Geometry check sheet. Reference: the model listing, model coordinates, mm. A direction names the side the tool comes from. Coordinates: 2 decimals unless noted, no trailing zeros. Write each loop counter-clockwise with the first axis right and the second up, starting at its lowest first coordinate (ties: lowest second). Pieces come first, ordered by that corner, then holes. Notation, with made-up numbers: (76.5, 87) -> (129.5, 87) arc R21 cw to (129.5, 124) -> close; hole circle Ø8 at (-22, 10.25). An arc over 180 degrees is marked (long way). Put each result on its own line as item: value. Start each with the question number.
from build123d import *

# Parameters (mm, degrees)
F0_W      = 15
F0_H      = 63
F1_DEPTH  = 40
F4_W      = 15
F4_H      = 60
F2_W      = 45
F2_H      = 80
F1_FACE_W = 45
F1_FACE_H = 80
F8_W      = 30
F8_H      = 30
F9_DEPTH  = 50


with BuildPart() as f1:
    # F0 (on Front) → F1 (new body, symmetric)
    with BuildSketch(Plane.XZ):
        Polygon((-52.5, -6), (52.5, -6), (52.5, 6), (37.5, 6), (-52.5, 6), align=None)
        with Locations((45, 37.5)):
            Rectangle(F0_W, F0_H)
    extrude(amount=F1_DEPTH, both=True)

    # F4 (on offset) → F5 section 0
    with BuildSketch(Plane.XY.offset(52)):
        with Locations((-27, 0)):
            Rectangle(F4_W, F4_H)
    # F2 (on face) → F5 section 1
    with BuildSketch(Plane.XY.offset(6)):
        with Locations((-30, 0)):
            Rectangle(F2_W, F2_H)
    loft()

    # F4 (on offset) → F6 section 0
    with BuildSketch(Plane.XY.offset(52)):
        with Locations((30, 0)):
            Rectangle(F4_W, F4_H)
    # F1_face (on face) → F6 section 1
    with BuildSketch(Plane(origin=(-7.5, 0, 6), x_dir=(1, 0, 0), z_dir=(0, 0, 1))):
        with Locations((22.5, 0)):
            Rectangle(F1_FACE_W, F1_FACE_H)
    loft()

    # F8 (on offset) → F9 (cut)
    with BuildSketch(Plane.YZ.offset(-52.5)):
        with Locations((0, 37)):
            Rectangle(F8_W, F8_H)
    extrude(amount=F9_DEPTH, mode=Mode.SUBTRACT)


solid = f1.part
Item 1: Section check B-B, the plane z = 59. Enter the section's corners in (x, y), and give its area (3 significant figures).
Item 2: Scan lines: line 1 along Z through (x, y) = (30.5, 27); line 2 along Y through (x, z) = (-24.5, 43); line 3 along X through (y, z) = (21.5, 25). Record each from-to range of solid material in increasing order. Write a range as [from, to].
Item 3: Access from +Z, -Z, +X, -X, +Y, -Y to the whole of each face (thin tool, end or side, straight path). Record for faces 4 (the flat face through (-29, -15, 33)), 5 (the flat face through (-1, -1, -6)), 6 (the flat face through (-27, -23, 52)).
Item 4: Go/stop test with flat-tipped pins: P1, Ø16.5, axis at x = -23.5, y = -26, coming from the +Z side; P2, Ø9, axis at x = -28, y = -7.5, coming from the +Z side; P3, Ø4, axis at x = 3.5, z = 11.5, coming from the -Y side; P4, Ø8, axis at x = -22, z = 56.5, coming from the +Y side. Record where each tip stops, or that it passes through.
Item 5: Mould release check, pull along Y, two halves, no side actions. Record for faces 1 (the flat face through (45, -1, 69)), 2 (the flat face through (-29, 0, 22)), 3 (the flat face through (15, -40, 4)): released by +Y, released by -Y, zero draft, split by the parting line, or undercut.
Item 6: Section check A-A, the plane z = 29. Give the number of separate pieces and of enclosed holes in the cut face, and give its area (3 significant figures).
From the geometry:
1. outline: (37.5, -40) -> (52.5, -40) -> (52.5, 40) -> (37.5, 40) -> close
1. area: 1,200 mm²
2. line 1: [-6, 52]
2. line 2: [-31.96, -15], [15, 31.96]
2. line 3: [-45.07, -12.46], [4.89, 52.5]
3. face 4: +Z, -X
3. face 5: -Z, +X, -X, +Y, -Y
3. face 6: +Z, -X, +Y, -Y
4. P1: z = 52
4. P2: z = 22
4. P3: y = -39.24
4. P4: through
5. face 1: zero draft
5. face 2: undercut
5. face 3: released by -Y
6. separate pieces: 3
6. enclosed holes: 0
6. area: 4,500 mm²
